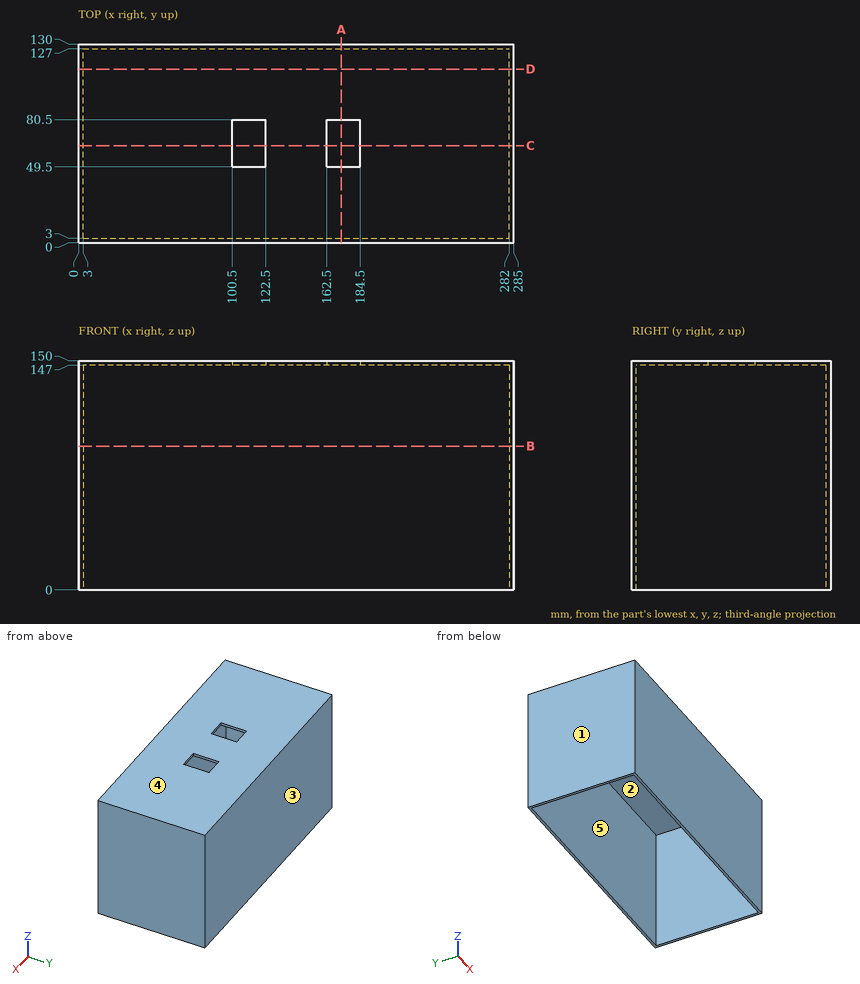
The drawing under review shows one solid part. Ordinate dimensions are in mm from its lowest x, y, z. A direction names the side the tool comes from. Round coordinates to 2 decimals unless told otherwise and drop trailing zeros. Loops run counter-clockwise (first coordinate to the right, second up) from the corner with the lowest first, then second, coordinate; pieces in that order, holes last. Notation, with made-up numbers: (11.5, 52.25) - (44.5, 52.25) arc R5 cw to (44.5, 58.25) - close; hole circle Ø10 at (89, -5.5). An arc over 180 degrees is marked (long way). Put each result on its own line as item: value. Start each with the question number.
1. Mouldability with a two-part tool opening along Y and no side actions: class the marked faces 3, 4 and 5 as +Y half, -Y half, draft (parallel to the pull), parting line (faces both ways), or undercut.
2. For the marked faces 1 and 2, list the 3-axis set-ups (+Z, -Z, +X, -X, +Y, -Y) from which the entire face can be reached by the end or side of a thin tool; tool diameter is ignored.
3. Consider section B-B on z = 94. State the section outline as (x, y) points, plus the area to 3 significant figures.
4. Insertion check: P1, Ø3.5, axis at x = 173.5, z = 148.5, coming from the -Y side; P2, Ø1, axis at x = 53, y = 77, coming from the -Z side. Each pin has a flat end and moves straight along its axis. Give the tip position at first contact, or say it passes through.
5. Consider section D-D on y = 113.5. State the section outline as (x, z) points.
6. Consider section A-A on x = 172. State the section outline as (y, z) points.
7. Consider section C-C on y = 63.5. State the section outline as (x, z) points.
8. For probe 1 along Y at (x, z) = (100, 112); probe 2 along X at (y, z) = (77, 137); probe 3 along Z at (x, y) = (135, 23.5), list the stretches that pass through material, from the lowest coordinate up. Write a range as [from, to].
Result sheet:
1. face 3: +Y half
1. face 4: draft
1. face 5: undercut
2. face 1: +Z, -Z, -X, +Y, -Y
2. face 2: -Z
3. outline: (0, 0) - (285, 0) - (285, 130) - (0, 130) - close; hole (3, 3) - (282, 3) - (282, 127) - (3, 127) - close
3. area: 2,450 mm^2
4. P1: y = 0
4. P2: z = 147
5. outline: (0, 0) - (3, 0) - (3, 147) - (282, 147) - (282, 0) - (285, 0) - (285, 150) - (0, 150) - close
6. outline: (0, 0) - (3, 0) - (3, 147) - (49.5, 147) - (49.5, 150) - (0, 150) - close; (80.5, 147) - (127, 147) - (127, 0) - (130, 0) - (130, 150) - (80.5, 150) - close
7. outline: (0, 0) - (3, 0) - (3, 147) - (100.5, 147) - (100.5, 150) - (0, 150) - close; (122.5, 147) - (162.5, 147) - (162.5, 150) - (122.5, 150) - close; (184.5, 147) - (282, 147) - (282, 0) - (285, 0) - (285, 150) - (184.5, 150) - close
8. probe 1: [0, 3], [127, 130]
8. probe 2: [0, 3], [282, 285]
8. probe 3: [147, 150]
